Geometry: see drawing. Coordinates: mm, zero at the bounding-box minimum. Give positions to 0.01 mm unless a question says otherwise; leave off trailing zeros. Write each loop counter-clockwise with the first axis right and the second up, starting at its lowest first coordinate (ties: lowest second). Pieces come first, ordered by that corner, then holes. Notation, with made-up numbers: (72, 69) -> (113, 69) arc R18 ccw to (113, 85) -> close; hole circle Ø4 at (79.5, 48.5). An arc over 180 degrees is marked (long way). Use CSV: the item, a comma, the result in double quotes. Start each with the question number.
1) Material intervals for line 1 (Z direction, x = 10, y = 1.3); line 2 (X direction, y = 1.2, z = 4); line 3 (X direction, y = 1.1, z = 34.5), sorted ascending. Write a range as [from, to].
2) Section C-C (x = 10). Output: boundary loops of the cut face in (y, z), plus the area to 3 significant figures.
3) Section B-B (y = 0.7). Output: boundary loops of the cut face in (x, z), plus the area to 3 significant figures.
4) Section A-A (z = 34.5). Output: boundary loops of the cut face in (x, y), plus the area to 3 significant figures.
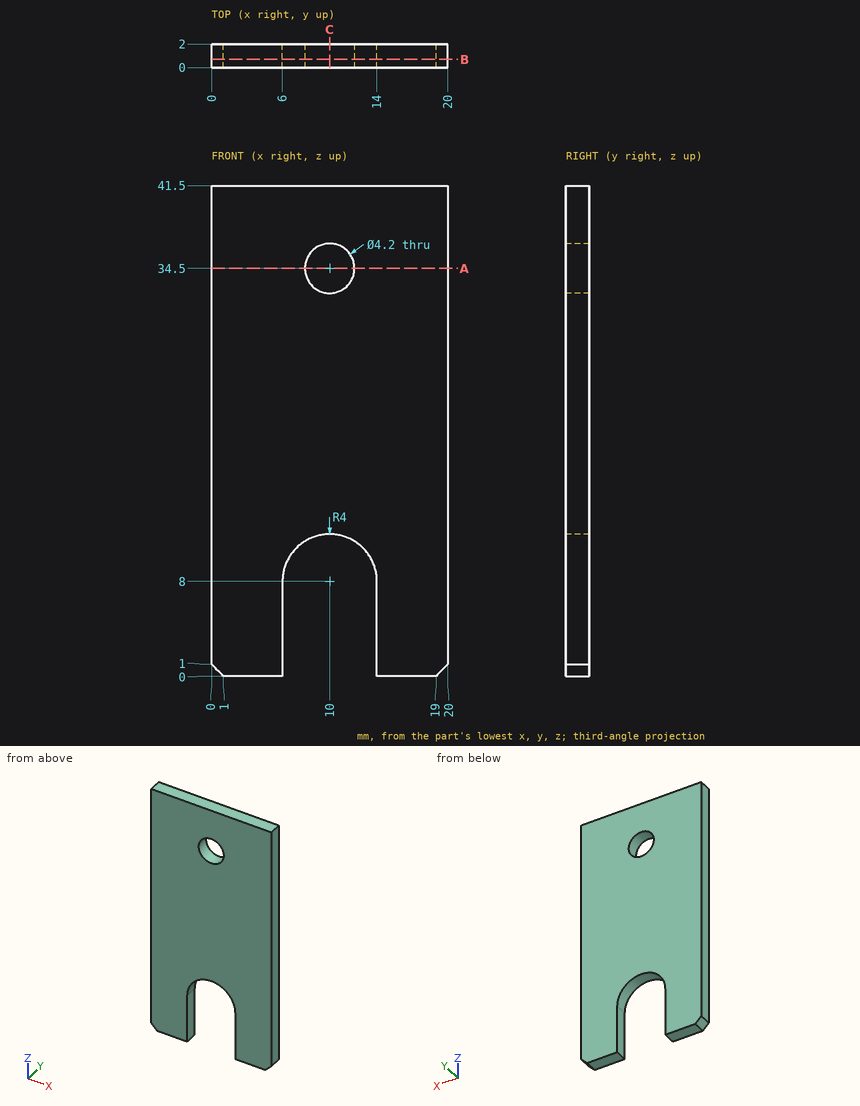
Answers follow:
1,line 1,"z = [12, 32.4], [36.6, 41.5]"
1,line 2,"x = [0, 6], [14, 20]"
1,line 3,"x = [0, 7.9], [12.1, 20]"
2,outline,"(0, 12) -> (2, 12) -> (2, 32.4) -> (0, 32.4) -> close; (0, 36.6) -> (2, 36.6) -> (2, 41.5) -> (0, 41.5) -> close"
2,area,"50.6 mm^2"
3,outline,"(0, 1) -> (1, 0) -> (6, 0) -> (6, 8) arc R4 cw to (14, 8) -> (14, 0) -> (19, 0) -> (20, 1) -> (20, 41.5) -> (0, 41.5) -> close; hole circle Ø4.2 at (10, 34.5)"
3,area,"726 mm^2"
4,outline,"(0, 0) -> (7.9, 0) -> (7.9, 2) -> (0, 2) -> close; (12.1, 0) -> (20, 0) -> (20, 2) -> (12.1, 2) -> close"
4,area,"31.6 mm^2"
